```python
from build123d import *

# Parameters (mm, degrees)
ESQUISSE3_W             = 1.75
ESQUISSE3_H             = 18.21482984
CHANFREIN1_SIZE         = 0.5
ESQUISSE6_R             = 2.5
ENL_V_MAT_EXTRU_1_DEPTH = 7.5


with BuildPart() as part:
    # Esquisse2 → Base-R_volution (revolve)
    with BuildSketch(Plane(origin=(0, 0, 0), x_dir=(0, 0, -1), z_dir=(1, 0, 0)), mode=Mode.PRIVATE) as base_r_volution_sk:
        Polygon((0, -3), (0, -6), (18, -6), (18, -8), (40, -8), (40, -5), (72.5, -5), (72.5, 0), (42.732050808, 0), (41, -3), align=None)
    revolve(base_r_volution_sk.sketch.rotate(Axis((0, 0, 0), (0, 0, 1)), 270), axis=Axis((0, 0, 0), (0, 0, 1)))

    # Esquisse3 → Enl_vement de mati_re-R_volution1 (revolve, cut)
    with BuildSketch(Plane(origin=(0, 0, -35), x_dir=(-1, 0, 0), z_dir=(0, 0, -1)), mode=Mode.PRIVATE) as enl_vement_de_mati_re_r_volution1_sk:
        with Locations((-0.875, 0.285598377)):
            Rectangle(ESQUISSE3_W, ESQUISSE3_H)
    revolve(enl_vement_de_mati_re_r_volution1_sk.sketch.rotate(Axis((0, 0, -35), (0, -1, 0)), 90), axis=Axis((0, 0, -35), (0, -1, 0)), mode=Mode.SUBTRACT)

    # Chanfrein1
    chanfrein1_edges = [part.edges().sort_by_distance(p)[0] for p in [
        (5, 0, -72.5),
    ]]
    chamfer(chanfrein1_edges, length=CHANFREIN1_SIZE)

    # Esquisse6 → Enl_v. mat.-Extru.1 (cut, symmetric)
    with BuildSketch(Plane(origin=(0, 0, 0), x_dir=(1, 0, 0), z_dir=(0, 1, 0))):
        with Locations(Location((0, 67.5, 0), (0, 0, 270))):
            Circle(ESQUISSE6_R)
    extrude(amount=ENL_V_MAT_EXTRU_1_DEPTH, both=True, mode=Mode.SUBTRACT)

    # Esquisse5 → Enl_vement de mati_re-R_volution3 (revolve, cut)
    with BuildSketch(Plane(origin=(0, 0, 0), x_dir=(0, 0, -1), z_dir=(1, 0, 0)), mode=Mode.PRIVATE) as enl_vement_de_mati_re_r_volution3_sk:
        Polygon((24.6, 30), (24.6, 5.4), (27.5, 5.4), (27.5, 20), (48, 20), (48, 3.36), (50, 3.36), (50, 30), align=None)
    revolve(enl_vement_de_mati_re_r_volution3_sk.sketch.rotate(Axis((0, 0, 18.428634536), (0, 0, -1)), 90), axis=Axis((0, 0, 18.428634536), (0, 0, -1)), mode=Mode.SUBTRACT)


solid = part.part
```
The model under review builds one solid part; all positions refer to its coordinate system, in mm. A direction names the side the tool comes from. Give positions to 0.01 mm unless a question says otherwise; leave off trailing zeros. Write each loop counter-clockwise with the first axis right and the second up, starting at its lowest first coordinate (ties: lowest second). Pieces come first, ordered by that corner, then holes.
(1) Tool access review of faces 4 (the flat face through (1.2, 3.3, -50)), 5 (the cylindrical face through (-1.735, 5.26, -35.228)), 6 (the cylindrical face through (-2.86, -0.9, -20.21)), 7 (the cylindrical face through (1.73, 7.81, -21.35)), 8 (the cylindrical face through (1.08, 4.88, -44.06)): name each direction out of +Z, -Z, +X, -X, +Y, -Y from which nothing blocks a thin tool from reaching the whole face with its end or side.
(2) The part is to be moulded in two halves that separate along Z. For faces 1 (the flat face through (0, 0, -72.5)), 2 (the flat face through (3.3, -1.2, -48)), 3 (the cylindrical face through (-5.723, -1.802, -9.126)), say which applies: released by +Z, released by -Z, zero draft, split by the parting line, or undercut.
(3) Consider section B-B, the plane z = -4.5. Give the boundary of the cut face in (x, y).
(4) Consider section A-A, the plane x = -6.75. Give the boundary of the cut face in (y, z).
(5) Consider section C-C, the plane z = -35. Give the boundary of the cut face in (x, y).
(6) For P1, Ø1, axis at y = 5, z = -45, coming from the +X side; P2, Ø3, axis at y = 3.5, z = -14.5, coming from the +X side, all flat-tipped, find the tip position at first contact; note any pin that passes through.
(7) To check wall thickness, follow L1, parallel to Z at x = 0.75, y = -5.5; L2, parallel to Z at x = 2.75, y = -5.75; L3, parallel to Y at x = 0, z = -11. State the ranges of each line that lie inside material, in increasing order.
(8) Consider section D-D, the plane z = -67.5. Give the boundary of the cut face in (x, y).
Returned:
1. face 4: none
1. face 5: +Y, -Y
1. face 6: +Z
1. face 7: +Z, -Z
1. face 8: -Z
2. face 1: released by -Z
2. face 2: undercut
2. face 3: zero draft
3. outline: circle Ø12 at (0, 0); hole circle Ø6 at (0, 0)
4. outline: (-4.29, -40) - (4.29, -40) - (4.29, -27.5) - (-4.29, -27.5) - close; (-4.29, -24.6) - (4.29, -24.6) - (4.29, -18) - (-4.29, -18) - close
5. outline: (-1.75, -7.81) - (-1.75, -2.44) arc R3 cw to (-1.75, 2.44) - (-1.75, 7.81) arc R8 ccw to start; (1.75, -7.81) arc R8 ccw to (1.75, 7.81) - (1.75, 2.44) arc R3 cw to (1.75, -2.44) - close
6. P1: stops at x = 2.18
6. P2: stops at x = 5.66
7. L1: z = -40 to -36.58, -33.42 to -27.5, -24.6 to 0
7. L2: z = -40 to -27.5, -24.6 to -18
7. L3: y = -6 to -3, 3 to 6
8. outline: (-2.5, -4.33) - (-2.5, 4.33) arc R5 ccw to start; (2.5, -4.33) arc R5 ccw to (2.5, 4.33) - close
